Part model, mm, in its own coordinate system. Round coordinates to 2 decimals unless told otherwise and drop trailing zeros. Loops run counter-clockwise (first coordinate to the right, second up) from the corner with the lowest first, then second, coordinate; pieces in that order, holes last. Notation, with made-up numbers: M 58.5,40.25 L 117.5,40.25 A17 cw 117.5,55.25 Z; hole C 78.5,75 d3. An arc over 180 degrees is marked long. Put each result on its own line as item: value. Start each with the question number.
```python
from build123d import *

# Parameters (mm, degrees)
SKETCH2_R           = 1.5
BOSS_EXTRUDE1_DEPTH = 4
CUT_EXTRUDE1_DEPTH  = 10
CUT_EXTRUDE2_DEPTH  = 10


with BuildPart() as part:
    # Sketch2 → Boss-Extrude1 (new body)
    with BuildSketch(Plane.XY):
        Polygon((-201.085, 510.519303279), (-148.79, -87.200696721), (148.79, -87.200696721), (201.085, 510.519303279), align=None)
        with Locations((-143.497000101, -21.490696721)):
            Circle(SKETCH2_R, mode=Mode.SUBTRACT)
        with Locations((-146.547451097, 13.376117712)):
            Circle(SKETCH2_R, mode=Mode.SUBTRACT)
        with Locations((-149.597902093, 48.242932145)):
            Circle(SKETCH2_R, mode=Mode.SUBTRACT)
        with Locations((-178.360333434, 376.989303279)):
            Circle(SKETCH2_R, mode=Mode.SUBTRACT)
        with Locations((-181.410784431, 411.856117712)):
            Circle(SKETCH2_R, mode=Mode.SUBTRACT)
        with Locations((-184.461235427, 446.722932145)):
            Circle(SKETCH2_R, mode=Mode.SUBTRACT)
        with Locations(Location((143.497000101, -21.490696721, 0), (0, 0, 180))):
            Circle(SKETCH2_R, mode=Mode.SUBTRACT)
        with Locations(Location((146.547451097, 13.376117712, 0), (0, 0, 180))):
            Circle(SKETCH2_R, mode=Mode.SUBTRACT)
        with Locations(Location((149.597902093, 48.242932145, 0), (0, 0, 180))):
            Circle(SKETCH2_R, mode=Mode.SUBTRACT)
        with Locations((180.519233461, 401.665041377)):
            Circle(SKETCH2_R, mode=Mode.SUBTRACT)
        with Locations((177.468708595, 366.798233406)):
            Circle(SKETCH2_R, mode=Mode.SUBTRACT)
        with Locations((174.418183729, 331.931425436)):
            Circle(SKETCH2_R, mode=Mode.SUBTRACT)
    extrude(amount=BOSS_EXTRUDE1_DEPTH)

    # Sketch4 → Cut-Extrude1 (cut)
    with BuildSketch(Plane.XY.offset(4)):
        Polygon((-34.094299882, 464.527144648), (-112.369249077, 383.780354951), (-132.143973084, 343.406960103), (-53.869023889, 424.153749799), align=None)
        Polygon((-0.812513571, 420.480908047), (-79.087462766, 339.73411835), (-98.862186773, 299.360723502), (-20.587237578, 380.107513199), align=None)
        Polygon((106.781302599, 457.941673616), (28.506353404, 377.19488392), (8.731629397, 336.821489072), (87.006578592, 417.568278768), align=None)
        Polygon((-12.949090157, 324.872537818), (-91.224039352, 244.125748122), (-110.99876336, 203.752353274), (-32.723814164, 284.49914297), align=None)
        Polygon((20.332696154, 280.826301217), (-57.942253041, 200.079511521), (-77.716977049, 159.706116673), (0.557972147, 240.452906369), align=None)
        Polygon((127.926512324, 318.287066787), (49.651563128, 237.54027709), (29.876839121, 197.166882242), (108.151788317, 277.913671939), align=None)
        Polygon((-3.521579741, 167.145743121), (-81.796528937, 86.398953425), (-101.571252944, 46.025558577), (-23.296303748, 126.772348273), align=None)
        Polygon((29.76020657, 123.09950652), (-48.514742626, 42.352716824), (-68.289466633, 1.979321976), (9.985482563, 82.726111672), align=None)
        Polygon((137.35402274, 160.560272089), (59.079073544, 79.813482393), (39.304349537, 39.440087545), (117.579298732, 120.186877241), align=None)
    extrude(amount=-CUT_EXTRUDE1_DEPTH, mode=Mode.SUBTRACT)

    # Sketch5 → Cut-Extrude2 (cut)
    with BuildSketch(Plane.XY.offset(4)):
        with BuildLine():
            Line((-79.098896029, -40.056454397), (82.394683364, -40.056454397))
            ThreePointArc((82.394683364, -40.056454397), (87.394683364, -45.056454397), (82.394683364, -50.056454397))
            Line((82.394683364, -50.056454397), (-79.098896029, -50.056454397))
            ThreePointArc((-79.098896029, -50.056454397), (-84.098896029, -45.056454397), (-79.098896029, -40.056454397))
        make_face()
    extrude(amount=-CUT_EXTRUDE2_DEPTH, mode=Mode.SUBTRACT)


solid = part.part
```
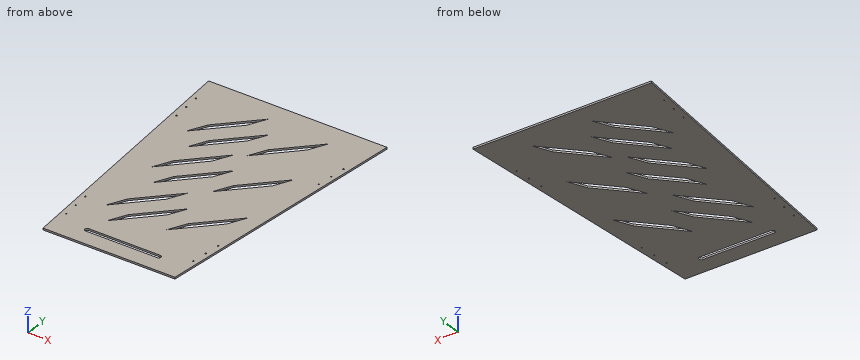
1. Cut at B-B, the plane y = 350. Give the cut face in (x, z).
2. Cut at D-D, the plane z = 1.55. Give the number of separate pieces and of enclosed holes in the cut face, and give its area (3 significant figures).
3. Cut at C-C, the plane y = -11. Give the cut face in (x, z).
4. Wall check: L1, parallel to X at y = 50.5, z = 2.4; L2, parallel to Y at x = -144, z = 3.6; L3, parallel to X at y = 385.5, z = 3.65. Give the ranges that are in metal, low to high.
5. Drop flat-ended pins along their axis: pin 1 (3.5 mm diameter, centred on x = -143.5, y = -21.49, fed in from +Z); pin 2 (1 mm diameter, centred on y = 136.5, z = 3.5, fed in from +X); pin 3 (2 mm diameter, centred on y = 416, z = 1.5, fed in from -X). Give the stop position or say it passes through.
6. Cut at A-A, the plane x = 76.5. Give the cut face in (y, z), and give its area (3 significant figures).
Results list:
1. outline: M -187.04,0 L -128.91,0 L -128.91,4 L -187.04,4 Z; M -125.75,0 L -69.14,0 L -69.14,4 L -125.75,4 Z; M -49.77,0 L 15.19,0 L 15.19,4 L -49.77,4 Z; M 21.51,0 L 187.04,0 L 187.04,4 L 21.51,4 Z
2. separate pieces: 1
2. enclosed holes: 22
2. area: 193,000 mm^2
3. outline: M -155.46,0 L 155.46,0 L 155.46,4 L -155.46,4 Z
4. L1: x = -160.84 to -99.38, -97.23 to -40.62, -21.25 to 44.72, 50.03 to 160.84
4. L2: y = -87.2 to -22.9, -20.08 to 510.52
4. L3: x = -190.15 to -110.7, -91.34 to -34.72, -17.95 to 36.56, 55.92 to 190.15
5. pin 1: stops at z = 4
5. pin 2: stops at x = 168.41
5. pin 3: stops at x = -192.9
6. outline: M -87.2,0 L -50.06,0 L -50.06,4 L -87.2,4 Z; M -40.06,0 L 77.81,0 L 77.81,4 L -40.06,4 Z; M 97.78,0 L 245.26,0 L 245.26,4 L 97.78,4 Z; M 265.24,0 L 406.73,0 L 406.73,4 L 265.24,4 Z; M 426.7,0 L 510.52,0 L 510.52,4 L 426.7,4 Z
6. area: 2,110 mm^2
